```python
from build123d import *

# Parameters (mm, degrees)
SKETCH1_W               = 25
SKETCH1_H               = 25
BOSS_EXTRUDE1_DEPTH     = 500
FILLET1_R               = 2
CUT_EXTRUDE1_DEPTH      = 1001.390548736
CUT_EXTRUDE1_DEPTH_BACK = 1001.390548736
SKETCH2_W               = 20.4
SKETCH2_H               = 20.4
FILLET2_R               = 2


with BuildPart() as part:
    # Sketch1 → Boss-Extrude1 (new, symmetric)
    with BuildSketch(Plane(origin=(0, 0, 0), x_dir=(0, 0, -1), z_dir=(1, 0, 0))):
        with Locations((0, 12.5)):
            Rectangle(SKETCH1_W, SKETCH1_H)
    extrude(amount=BOSS_EXTRUDE1_DEPTH, both=True)

    # Fillet1
    fillet1_edges = [part.edges().sort_by_distance(p)[0] for p in [
        (0, 25, 12.5),
        (0, 25, -12.5),
        (0, 0, -12.5),
        (0, 0, 12.5),
    ]]
    fillet(fillet1_edges, radius=FILLET1_R)

    # Sketch2 → Cut-Extrude1 (cut, two sides: drawn at the far end of the back side and taken through both)
    with BuildSketch(Plane(origin=(500, 0, 0), x_dir=(0, 0, -1), z_dir=(1, 0, 0)).offset(-CUT_EXTRUDE1_DEPTH_BACK)):
        with Locations((0, 12.5)):
            Rectangle(SKETCH2_W, SKETCH2_H)
    extrude(amount=CUT_EXTRUDE1_DEPTH + CUT_EXTRUDE1_DEPTH_BACK, mode=Mode.SUBTRACT)

    # Fillet2
    fillet2_edges = [part.edges().sort_by_distance(p)[0] for p in [
        (0, 22.7, 10.2),
        (0, 22.7, -10.2),
        (0, 2.3, -10.2),
        (0, 2.3, 10.2),
    ]]
    fillet(fillet2_edges, radius=FILLET2_R)


solid = part.part
```
Geometry check sheet. Reference: the model listing, model coordinates, mm. A direction names the side the tool comes from. Round coordinates to 2 decimals unless told otherwise and drop trailing zeros. Order: outer loops, then holes, each group sorted by start corner. A loop starts at its lowest first (then second) coordinate and runs counter-clockwise, first axis right, second up. Notation, with made-up numbers: M -15,-27.75 L 5,-27.75 A18 cw 5,1.25 Z; hole C 63,72.5 d1. An arc over 180 degrees is marked long. Answer as CSV lines item,"result".
1) Thickness scan on probe 1 along Y at (x, z) = (-79.5, 3.75); probe 2 along Z at (x, y) = (-436, 15.5); probe 3 along Z at (x, y) = (-358, 2.75). Record the ranges inside material, lowest first. Write a range as [from, to].
Entries:
probe 1,"[0, 2.3], [22.7, 25]"
probe 2,"[-12.5, -10.2], [10.2, 12.5]"
probe 3,"[-12.5, -9.46], [9.46, 12.5]"
2) Gauge pin test, flat end, axial feed: pin 1 Ø1 at (y, z) = (6.5, -9.5) entering from +X. Record the tip position at first contact, or that the pin passes through.
Entries:
pin 1,"through"
3) Mould release check, pull along Z, two halves, no side actions. Record for faces 3 (the face through (-7, 22.7, 0)), 4 (the face through (7, 12, -12.5)), 5 (the face through (500, 13, 11)), 6 (the face through (7, 12, 12.5)): +Z half, -Z half, draft (parallel to the pull), parting line (faces both ways), or undercut.
Entries:
face 3,"undercut"
face 4,"-Z half"
face 5,"draft"
face 6,"+Z half"
4) Sectioned sample at C-C on x = -202. Record the cut outline in (y, z).
Entries:
outline,"M 0,-10.5 A2 ccw 2,-12.5 L 23,-12.5 A2 ccw 25,-10.5 L 25,10.5 A2 ccw 23,12.5 L 2,12.5 A2 ccw 0,10.5 Z; hole M 2.3,-8.2 A2 ccw 4.3,-10.2 L 20.7,-10.2 A2 ccw 22.7,-8.2 L 22.7,8.2 A2 ccw 20.7,10.2 L 4.3,10.2 A2 ccw 2.3,8.2 Z"
5) Sectioned sample at A-A on y = 9.25. Record the cut outline in (x, z), and give its area (3 significant figures).
Entries:
outline,"M -500,-12.5 L 500,-12.5 L 500,-10.2 L -500,-10.2 Z; M -500,10.2 L 500,10.2 L 500,12.5 L -500,12.5 Z"
area,"4,600 mm2"
6) Sectioned sample at B-B on z = -1. Record the cut outline in (x, y).
Entries:
outline,"M -500,0 L 500,0 L 500,2.3 L -500,2.3 Z; M -500,22.7 L 500,22.7 L 500,25 L -500,25 Z"
7) Tool access check on faces 1 (the face through (-7, 12, -10.2)), 2 (the face through (7, 0, 0)). Record the directions out of +Z, -Z, +X, -X, +Y, -Y that give a thin tool (end or side, any length) a straight path to the whole face; none if there is none.
Entries:
face 1,"+X, -X"
face 2,"+Z, -Z, +X, -X, -Y"
